from build123d import *

# Parameters (mm, degrees)
EXTRUDE_1_DEPTH          = 42
SKETCH_2_R               = 9
CUT_EXTRUDE_1_DEPTH      = 178.330200474
SKETCH_3_W               = 50
SKETCH_3_H               = 49
CUT_EXTRUDE_2_DEPTH      = 30
SKETCH_4_W               = 20
SKETCH_4_H               = 71
CUT_EXTRUDE_3_DEPTH      = 182.022098099
CUT_EXTRUDE_START        = -3
SKETCH_5_R               = 11.05
CUT_EXTRUDE_4_DEPTH      = 10
FILLET_1_R               = 3
FILLET_2_R               = 3
SKETCH_6_R               = 7.5
CUT_EXTRUDE_5_DEPTH      = 10
SKETCH_8_R               = 1.65
CUT_EXTRUDE_6_DEPTH      = 175.877099799
SKETCH_9_R               = 4
CUT_EXTRUDE_7_DEPTH      = 3
CUT_EXTRUDE_8_DEPTH      = 178.330200582
CUT_EXTRUDE_8_DEPTH_BACK = 178.330200582
SKETCH_14_R              = 15.1
CUT_EXTRUDE_9_DEPTH      = 10
SKETCH_15_R              = 11.1
CUT_EXTRUDE_10_DEPTH     = 2.1


with BuildPart() as part:
    # 草图1 → 凸台-拉伸1 (new body)
    with BuildSketch(Plane.XY):
        with BuildLine():
            Line((-21, 0), (-21, 150))
            ThreePointArc((-21, 150), (0, 171), (21, 150))
            Line((21, 150), (21, 0))
            ThreePointArc((21, 0), (0, -21), (-21, 0))
        make_face()
    extrude(amount=EXTRUDE_1_DEPTH)

    # 草图2 → 切除-拉伸1 (cut, through all)
    with BuildSketch(Plane(origin=(0, 0, 0), x_dir=(-1, 0, 0), z_dir=(0, 0, -1))):
        with Locations((0, 50)):
            Circle(SKETCH_2_R)
    extrude(amount=-CUT_EXTRUDE_1_DEPTH, mode=Mode.SUBTRACT)

    # 草图3 → 切除-拉伸2 (cut)
    with BuildSketch(Plane(origin=(0, 0, 0), x_dir=(-1, 0, 0), z_dir=(0, 0, -1))):
        with Locations((0, 50)):
            Rectangle(SKETCH_3_W, SKETCH_3_H)
    extrude(amount=-CUT_EXTRUDE_2_DEPTH, mode=Mode.SUBTRACT)

    # 草图4 → 切除-拉伸3 (cut, through all)
    with BuildSketch(Plane.ZY.offset(21)):
        with Locations((21, 150)):
            Rectangle(SKETCH_4_W, SKETCH_4_H)
    extrude(amount=-CUT_EXTRUDE_3_DEPTH, mode=Mode.SUBTRACT)

    # 草图5 → 切除-拉伸4 (cut)
    with BuildSketch(Plane.XY.offset(42).offset(CUT_EXTRUDE_START)):
        with Locations((0, 150)):
            Circle(SKETCH_5_R)
    cut_extrude_4 = extrude(amount=-CUT_EXTRUDE_4_DEPTH, mode=Mode.SUBTRACT)

    # 圆角1
    fillet_1_edges = [part.edges().sort_by_distance(p)[0] for p in [
        (0, 171, 42),
        (-21, 75, 42),
        (0, -21, 42),
        (21, 75, 42),
    ]]
    fillet(fillet_1_edges, radius=FILLET_1_R)

    # 圆角2
    fillet_2_edges = [part.edges().sort_by_distance(p)[0] for p in [
        (-21, 12.75, 0),
        (21, 112.25, 0),
        (0, 25.5, 0),
        (0, 74.5, 0),
        (-21, 112.25, 0),
        (0, 171, 0),
        (21, 12.75, 0),
        (0, -21, 0),
    ]]
    fillet(fillet_2_edges, radius=FILLET_2_R)

    # 草图6 → 切除-拉伸5 (cut)
    with BuildSketch(Plane(origin=(0, 0, 39), x_dir=(-1, 0, 0), z_dir=(0, 0, -1))):
        with Locations((0, 150)):
            Circle(SKETCH_6_R)
    cut_extrude_5 = extrude(amount=-CUT_EXTRUDE_5_DEPTH, mode=Mode.SUBTRACT)

    # 镜向1: 切除-拉伸4, 切除-拉伸5 across plane
    add(cut_extrude_4.mirror(Plane.XY.offset(21)), mode=Mode.SUBTRACT)
    add(cut_extrude_5.mirror(Plane.XY.offset(21)), mode=Mode.SUBTRACT)

    # 草图8 → 切除-拉伸6 (cut, through all)
    with BuildSketch(Plane(origin=(0, 0, 30), x_dir=(-1, 0, 0), z_dir=(0, 0, -1))):
        with Locations((-15.5, 34.5)):
            Circle(SKETCH_8_R)
        with Locations((-15.5, 65.5)):
            Circle(SKETCH_8_R)
        with Locations((15.833547664, 65.5)):
            Circle(SKETCH_8_R)
        with Locations((15.5, 34.5)):
            Circle(SKETCH_8_R)
    extrude(amount=-CUT_EXTRUDE_6_DEPTH, mode=Mode.SUBTRACT)

    # 草图9 → 切除-拉伸7 (cut)
    with BuildSketch(Plane.XY.offset(42)):
        with Locations((15.5, 65.5)):
            Circle(SKETCH_9_R)
        with Locations((15.5, 34.5)):
            Circle(SKETCH_9_R)
        with Locations((-15.5, 65.5)):
            Circle(SKETCH_9_R)
        with Locations((-15.5, 34.5)):
            Circle(SKETCH_9_R)
    extrude(amount=-CUT_EXTRUDE_7_DEPTH, mode=Mode.SUBTRACT)

    # 草图13 → 切除-拉伸8 (cut, two sides: drawn at the far end of the back side and taken through both)
    with BuildSketch(Plane.XY.offset(42).offset(-CUT_EXTRUDE_8_DEPTH_BACK)):
        with BuildLine():
            ThreePointArc((6.6, 3.868139087), (3.803369295, 6.637535839), (0, 7.65))
            Line((0, 7.65), (0, -7.65))
            ThreePointArc((0, -7.65), (3.803369295, -6.637535839), (6.6, -3.868139087))
            Line((6.6, -3.868139087), (6.6, 3.868139087))
        make_face()
        with BuildLine():
            Line((0, -7.65), (0, 7.65))
            ThreePointArc((0, 7.65), (-7.65, 0), (0, -7.65))
        make_face()
    extrude(amount=CUT_EXTRUDE_8_DEPTH + CUT_EXTRUDE_8_DEPTH_BACK, mode=Mode.SUBTRACT)

    # 草图14 → 切除-拉伸9 (cut)
    with BuildSketch(Plane(origin=(0, 0, 0), x_dir=(-1, 0, 0), z_dir=(0, 0, -1))):
        Circle(SKETCH_14_R)
    extrude(amount=-CUT_EXTRUDE_9_DEPTH, mode=Mode.SUBTRACT)

    # 草图15 → 切除-拉伸10 (cut)
    with BuildSketch(Plane(origin=(0, 0, 30), x_dir=(-1, 0, 0), z_dir=(0, 0, -1))):
        with Locations((0, 50)):
            Circle(SKETCH_15_R)
    extrude(amount=-CUT_EXTRUDE_10_DEPTH, mode=Mode.SUBTRACT)


solid = part.part
The model under review builds one solid part; all positions refer to its coordinate system, in mm. A direction names the side the tool comes from. Give positions to 0.01 mm unless a question says otherwise; leave off trailing zeros. Loops run counter-clockwise (first coordinate to the right, second up) from the corner with the lowest first, then second, coordinate; pieces in that order, holes last. Notation, with made-up numbers: (39.25, 48) -> (46.25, 48) arc R8 cw to (46.25, 57) -> close; hole circle Ø6 at (9, 30). An arc over 180 degrees is marked (long way). Put each result on its own line as item: value. Start each with the question number.
1. We need section D-D on x = 3.5. State how many separate pieces and enclosed holes the cut face has, then the cut area to 3 significant figures.
2. We need section C-C on y = 34.5. State the section outline as (x, z) points.
3. We need section A-A on z = 27. State the section outline as (x, y) points, then the cut area to 3 significant figures.
4. Wall thickness on probe 1 along X at (y, z) = (65.5, 32); probe 2 along Z at (x, y) = (-10, 148.5); probe 3 along Y at (x, z) = (3, 29): over which ranges is each line inside the solid? List them lowest first.
5. We need section B-B on y = 132. State the section outline as (x, z) points, then the cut area to 3 significant figures.
6. For faces 1 (the face through (6.6, 0, 26)), 2 (the face through (0, 74.5, 16)), 3 (the face through (11.504, 65.676, 40.521)), list the 3-axis set-ups (+Z, -Z, +X, -X, +Y, -Y) from which the entire face can be reached by the end or side of a thin tool; tool diameter is ignored.
7. Mouldability with a two-part tool opening along Z and no side actions: class faces 4 (the face through (0.976, 157.436, 40.479)), 5 (the face through (7.2, 152.6, 39)), 6 (the face through (0, 76, 42)) as released by +Z, released by -Z, zero draft, split by the parting line, or undercut.
8. Clearance check with flat-ended pins moving along their axes: P1, Ø5, axis at x = -12, z = 18, coming from the -Y side; P2, Ø5, axis at x = -15.5, y = 65.5, coming from the -Z side; P3, Ø4, axis at x = 15, z = 6, coming from the -Y side. State where each tip first meets the part, or that it passes through.
Determined:
1. separate pieces: 5
1. enclosed holes: 0
1. area: 4,080 mm^2
2. outline: (-21, 30) -> (-17.15, 30) -> (-17.15, 39) -> (-19.5, 39) -> (-19.5, 41.6) arc R3 ccw to (-21, 39) -> close; (-13.85, 30) -> (13.85, 30) -> (13.85, 39) -> (11.5, 39) -> (11.5, 42) -> (-11.5, 42) -> (-11.5, 39) -> (-13.85, 39) -> close; (17.15, 30) -> (21, 30) -> (21, 39) arc R3 ccw to (19.5, 41.6) -> (19.5, 39) -> (17.15, 39) -> close
3. outline: (-21, 0) arc R21 ccw to (21, 0) -> (21, 25.5) -> (-21, 25.5) -> close; (-21, 74.5) -> (21, 74.5) -> (21, 114.5) -> (-21, 114.5) -> close; hole (6.6, -3.87) -> (6.6, 3.87) arc R7.65 ccw (long way) to start
3. area: 3,270 mm^2
4. probe 1: -21 to -17.48, -14.18 to 13.85, 17.15 to 21
4. probe 2: 0 to 3, 39 to 42
4. probe 3: -20.78 to -7.04, 7.04 to 25.5, 74.5 to 114.5
5. outline: (-21, 3) arc R3 ccw to (-18, 0) -> (18, 0) arc R3 ccw to (21, 3) -> (21, 11) -> (-21, 11) -> close; (-21, 31) -> (21, 31) -> (21, 39) arc R3 ccw to (18, 42) -> (-18, 42) arc R3 ccw to (-21, 39) -> close
5. area: 916 mm^2
6. face 1: +Z, -Z
6. face 2: -Z, +X, -X
6. face 3: +Z
7. face 4: zero draft
7. face 5: undercut
7. face 6: released by +Z
8. P1: y = -18.73
8. P2: z = 30
8. P3: y = -16.49
